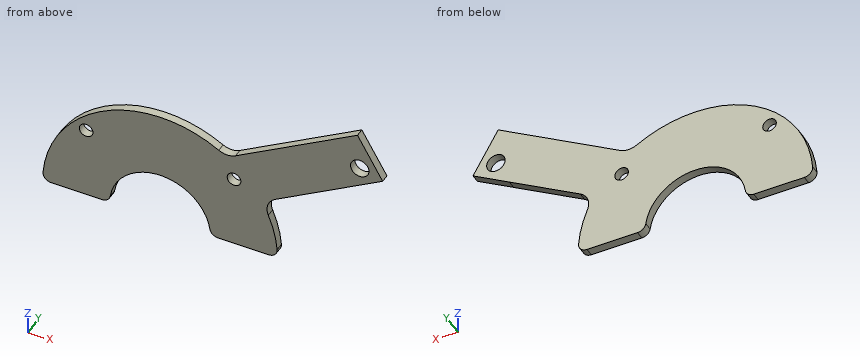
```python
from build123d import *

# Parameters (mm, degrees)
F1_DEPTH = 6.35
F3_D     = 10.3124
F4_R     = 12.7
F5_R     = 6.35
F7_D     = 14


# Not quite as in the source:
# - a feature names something its author has since deleted; it is built from what else it names


with BuildPart() as f1:
    # F0 (on Front) → F1 (new body)
    with BuildSketch(Plane.XZ):
        with BuildLine():
            Line((38.1, 0), (88.9, 0))
            ThreePointArc((88.9, 0), (85.8708059571, 23.0090131096), (76.9896583964, 44.45))
            Line((76.9896583964, 44.45), (141.0511618856, 81.4359262841))
            Line((141.0511618856, 81.4359262841), (168.5474684557, 97.3109262841))
            Line((168.5474684557, 97.3109262841), (149.4974684557, 130.3064941683))
            Line((149.4974684557, 130.3064941683), (122.0011618856, 114.4314941683))
            Line((122.0011618856, 114.4314941683), (50.5107648032, 73.1564941683))
            ThreePointArc((50.5107648032, 73.1564941683), (-41.3086129578, 78.7198100576), (-88.9, 0))
            Line((-88.9, 0), (-38.1, 0))
            ThreePointArc((-38.1, 0), (0, 38.1), (38.1, 0))
        make_face()
    extrude(amount=F1_DEPTH)

    # F3 (through all)
    with Locations(Plane.XZ.offset(6.35)):
        with Locations((-55.9918969149, 55.9918969149), (55.9918969149, 55.9918969149)):
            Hole(F3_D / 2)

    # F4
    f4_edges = [f1.edges().sort_by_distance(p)[0] for p in [
        (50.510765, -3.175, 73.156494),
        (76.989658, -3.175, 44.45),
    ]]
    fillet(f4_edges, radius=F4_R)

    # F5
    f5_edges = [f1.edges().sort_by_distance(p)[0] for p in [
        (88.9, -3.175, 0),
        (38.1, -3.175, 0),
        (-38.1, -3.175, 0),
        (-88.9, -3.175, 0),
    ]]
    fillet(f5_edges, radius=F5_R)

    # F7 (through all)
    with Locations(Plane.XZ.offset(6.35)):
        with Locations((151.1989458277, 101.9594489122)):
            Hole(F7_D / 2)


solid = f1.part
```
Input: part model. Units: mm. Frame: model coordinates. Give positions to 0.01 mm unless a question says otherwise; leave off trailing zeros. Write each loop counter-clockwise with the first axis right and the second up, starting at its lowest first coordinate (ties: lowest second). Pieces come first, ordered by that corner, then holes. Notation, with made-up numbers: (4.25, 51.5) - (37.25, 51.5) arc R21 ccw to (37.25, 63.5) - close; hole circle Ø6 at (-15.75, 78). An arc over 180 degrees is marked (long way). Write item = value, one per line. Start each with the question number.
1) Cut plane B-B (z = 29.5). Return loops of the section in (x, y), and give its area (3 significant figures).
2) Pin query (flat end, axial travel): pin 1 (1.5 mm diameter, centred on y = -5, z = 43, fed in from -X); pin 2 (2 mm diameter, centred on x = 75, y = -5, fed in from +Z); pin 3 (1 mm diameter, centred on y = -1, z = 82.5, fed in from +X). Return the tip coordinate at first contact, or that it passes through.
3) Material intervals for L1, parallel to Z at x = -77, y = -5.75; L2, parallel to X at y = -1, z = 78.5; L3, parallel to Z at x = 4, y = -0.5, sorted ascending. Write a range as [from, to].
4) Cut plane A-A (x = -55.5). Return loops of the section in (y, z).
5) Cut plane D-D (x = 77). Return loops of the section in (y, z).
6) Cut plane C-C (y = -2.75). Return loops of the section in (x, z).
Answers follow:
q1.outline = (-83.86, -6.35) - (-24.11, -6.35) - (-24.11, 0) - (-83.86, 0) - close; (24.11, -6.35) - (83.86, -6.35) - (83.86, 0) - (24.11, 0) - close
q1.area = 759 mm^2
q2.pin_1 = -78.22
q2.pin_2 = 87.87
q2.pin_3 = 143.76
q3.L1 = [0, 44.43]
q3.L2 = [-41.72, 41.72], [59.77, 135.97]
q3.L3 = [37.89, 88.81]
q4.outline = (-6.35, 0) - (0, 0) - (0, 50.86) - (-6.35, 50.86) - close; (-6.35, 61.12) - (0, 61.12) - (0, 69.45) - (-6.35, 69.45) - close
q5.outline = (-6.35, 0) - (0, 0) - (0, 88.45) - (-6.35, 88.45) - close
q6.outline = (-88.64, 6.84) arc R6.35 ccw to (-82.31, 0) - (-43.99, 0) arc R6.35 ccw to (-37.71, 5.44) arc R38.1 cw to (37.71, 5.44) arc R6.35 ccw to (43.99, 0) - (82.31, 0) arc R6.35 ccw to (88.64, 6.84) arc R88.9 ccw to (81.94, 34.48) arc R12.7 cw to (87.3, 50.4) - (168.55, 97.31) - (149.5, 130.31) - (57.15, 76.99) arc R12.7 cw to (44.45, 76.99) arc R88.9 ccw to start; hole circle Ø10.31 at (-55.99, 55.99); hole circle Ø10.31 at (55.99, 55.99); hole circle Ø14 at (151.2, 101.96)
